Can you work these out from the model? Positions are in its coordinate system, mm. A direction names the side the tool comes from. Round coordinates to 2 decimals unless told otherwise and drop trailing zeros. Write each loop counter-clockwise with the first axis right and the second up, starting at its lowest first coordinate (ties: lowest second). Pieces come first, ordered by that corner, then holes. Notation, with made-up numbers: (-19, 68) -> (-1, 68) arc R25 cw to (-1, 107) -> close; hole circle Ø9 at (43, 62.25). An arc over 180 degrees is marked (long way). Use CSV: the item, a comma, the result in double quotes.
```python
from build123d import *

# Parameters (mm, degrees)
BASE_FLANGE1_DEPTH = 1
EDGE_FLANGE2_DEPTH = 42.5


# Sheet-metal steps are written as plain solids
with BuildPart() as part:
    # Sketch1 → Base-Flange1 (new body)
    with BuildSketch(Plane.XY):
        with BuildLine():
            Line((-16, 0), (-16, -84))
            Line((-16, -84), (25, -84))
            Line((25, -84), (25, -40.5))
            ThreePointArc((25, -40.5), (25.146446609, -40.146446609), (25.5, -40))
            Line((25.5, -40), (84, -40))
            Line((84, -40), (84, 16))
            Line((84, 16), (0, 16))
            ThreePointArc((0, 16), (-11.313708499, 11.313708499), (-16, 0))
        make_face()
    extrude(amount=-BASE_FLANGE1_DEPTH)

    # Edge-Flange2 section (across the edge) → Edge-Flange2 (add)
    with BuildSketch(Plane(origin=(26, -41.5, -1), x_dir=(-1, 0, 0), z_dir=(0, -1, 0))):
        with BuildLine():
            Line((-1, 1), (-1, 14))
            Line((-1, 14), (0, 14))
            Line((0, 14), (0, 1))
            ThreePointArc((0, 1), (0.292893219, 0.292893219), (1, 0))
            Line((1, 0), (1, -1))
            ThreePointArc((1, -1), (-0.414213562, -0.414213562), (-1, 1))
        make_face()
    extrude(amount=EDGE_FLANGE2_DEPTH)


solid = part.part
```
Q1. Suppose I cut it at C-C (z = -12.5). Write out the boundary of the cut face in (x, y), and give its area (3 significant figures).
Resolved:
outline,"(26, -84) -> (27, -84) -> (27, -41.5) -> (26, -41.5) -> close"
area,"42.5 mm^2"
Q2. On a 3-axis mill with a long thin cutter (end or side, diameter ignored), from which of +Z, -Z, +X, -X, +Y, -Y can I reach the whole of each face in a straight line? I mean faces 1 (the face through (26, -62, -9)), 2 (the face through (-11.189, 11.437, -0.493)). Say none if no direction works.
Resolved:
face 1,"-Z, -X, +Y, -Y"
face 2,"+Z, -Z, -X, +Y"
Q3. Will these pins go through, and if not, where does the flat tip stop? P1, Ø4, axis at y = -54.5, z = -10, coming from the +X side; P2, Ø1.5, axis at y = -58, z = -9, coming from the -X side; P3, Ø1, axis at x = 26, z = -8, coming from the +Y side.
Resolved:
P1,"stops at x = 27"
P2,"stops at x = 26"
P3,"stops at y = -41.5"
Q4. Suppose I cut it at B-B (x = 62). Write out the boundary of the cut face in (y, z).
Resolved:
outline,"(-40, -1) -> (16, -1) -> (16, 0) -> (-40, 0) -> close"
Q5. Suppose I cut it at A-A (y = -47.5). Write out the boundary of the cut face in (x, z).
Resolved:
outline,"(-16, -1) -> (25, -1) arc R1 cw to (26, -2) -> (26, -15) -> (27, -15) -> (27, -2) arc R2 ccw to (25, 0) -> (-16, 0) -> close"
Q6. Please list where these lines run through material, in increasing order: probe 1 along Z at (x, y) = (0, -28.5); probe 2 along X at (y, z) = (-43.5, -9.75); probe 3 along Y at (x, z) = (66, -0.75).
Resolved:
probe 1,"z = -1 to 0"
probe 2,"x = 26 to 27"
probe 3,"y = -40 to 16"
